The model under review builds one solid part; all positions refer to its coordinate system, in mm. Round coordinates to 2 decimals unless told otherwise and drop trailing zeros. Loops run counter-clockwise (first coordinate to the right, second up) from the corner with the lowest first, then second, coordinate; pieces in that order, holes last. Notation, with made-up numbers: (32.5, 26.25) - (67.5, 26.25) arc R20 ccw to (67.5, 62.25) - close; hole circle Ø7 at (-21, -32.75). An arc over 180 degrees is marked (long way). Answer as CSV lines item,"result".
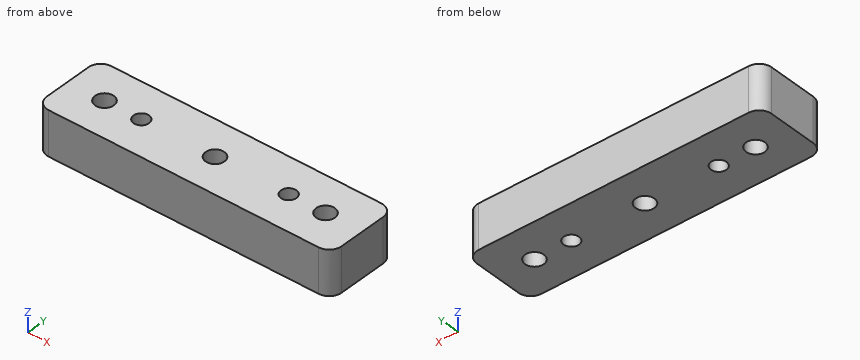
from build123d import *

# Parameters (mm, degrees)
BOSS_EXTRUDE1_DEPTH   = 12
SKETCH3_R             = 2.55
CUT_EXTRUDE2_DEPTH    = 43.941821107
M5X0_8_TAPPED_HOLE1_D = 4.2


with BuildPart() as part:
    # Sketch1 → Boss-Extrude1 (new body)
    with BuildSketch(Plane.XY):
        with BuildLine():
            Line((36.64, -10), (-36.64, -10))
            ThreePointArc((-36.64, -10), (-39.015878785, -9.015878785), (-40, -6.64))
            Line((-40, -6.64), (-40, 6.64))
            ThreePointArc((-40, 6.64), (-39.015878785, 9.015878785), (-36.64, 10))
            Line((-36.64, 10), (36.64, 10))
            ThreePointArc((36.64, 10), (39.015878785, 9.015878785), (40, 6.64))
            Line((40, 6.64), (40, -6.64))
            ThreePointArc((40, -6.64), (39.015878785, -9.015878785), (36.64, -10))
        make_face()
    extrude(amount=BOSS_EXTRUDE1_DEPTH)

    # Sketch3 → Cut-Extrude2 (cut, through all)
    with BuildSketch(Plane.XY.offset(12)):
        with Locations((-30, 0)):
            Circle(SKETCH3_R)
        with Locations(Location((30, 0, 0), (0, 0, 180))):
            Circle(SKETCH3_R)
        Circle(SKETCH3_R)
    extrude(amount=-CUT_EXTRUDE2_DEPTH, mode=Mode.SUBTRACT)

    # M5x0.8 Tapped Hole1 (through all)
    with Locations(Plane.XY.offset(12)):
        with Locations((-20, 0), (20, 0)):
            Hole(M5X0_8_TAPPED_HOLE1_D / 2)


solid = part.part
1. Clearance check with a flat-ended pin moving along its axis: pin 1 (3 mm diameter, centred on x = -30.5, y = -6.5, fed in from -Z). State where the tip first meets the part, or that it passes through.
Numbers:
pin 1,"stops at z = 0"
2. Take a section at A-A (x = -30). State the section outline as (y, z) points.
Numbers:
outline,"(-10, 0) - (-2.55, 0) - (-2.55, 12) - (-10, 12) - close; (2.55, 0) - (10, 0) - (10, 12) - (2.55, 12) - close"
3. Take a section at C-C (x = 1.5). State the section outline as (y, z) points, plus the area to 3 significant figures.
Numbers:
outline,"(-10, 0) - (-2.06, 0) - (-2.06, 12) - (-10, 12) - close; (2.06, 0) - (10, 0) - (10, 12) - (2.06, 12) - close"
area,"191 mm²"
4. Take a section at B-B (z = 1.75). State the section outline as (x, y) points, plus the area to 3 significant figures.
Numbers:
outline,"(-40, -6.64) arc R3.36 ccw to (-36.64, -10) - (36.64, -10) arc R3.36 ccw to (40, -6.64) - (40, 6.64) arc R3.36 ccw to (36.64, 10) - (-36.64, 10) arc R3.36 ccw to (-40, 6.64) - close; hole circle Ø5.1 at (-30, 0); hole circle Ø4.2 at (-20, 0); hole circle Ø5.1 at (0, 0); hole circle Ø4.2 at (20, 0); hole circle Ø5.1 at (30, 0)"
area,"1,500 mm²"
5. Wall thickness on probe 1 along Y at (x, z) = (20, 6.5); probe 2 along Y at (x, z) = (30, 9.25); probe 3 along X at (y, z) = (9, 11.5): over which ranges is each line inside the solid? List them lowest first.
Numbers:
probe 1,"y = -10 to -2.1, 2.1 to 10"
probe 2,"y = -10 to -2.55, 2.55 to 10"
probe 3,"x = -39.03 to 39.03"
